from build123d import *

# Parameters (mm, degrees)
BOSS_EXTRUDE1_DEPTH     = 7.75
CUT_EXTRUDE_THIN1_DEPTH = 42.810913647
CUT_EXTRUDE1_REACH      = 43.811
SKETCH3_W               = 7.8
SKETCH3_H               = 2.7
CHAMFER1_SIZE           = 0.5


with BuildPart() as part:
    # Sketch1 → Boss-Extrude1 (new, symmetric)
    with BuildSketch(Plane(origin=(0, 0, 0), x_dir=(0, 0, -1), z_dir=(1, 0, 0))):
        Polygon((0, 0), (40.3, 0), (40.3, 8), (38.3, 8), (38.3, 3.5), (19, 3.5), (19, 1.7), (14, 1.7), (14, 3.5), (9.6, 3.5), (9.6, 2.5), (3, 2.5), (3, 5.2), (1, 5.2), (1, 6.7), (0, 6.7), align=None)
    extrude(amount=BOSS_EXTRUDE1_DEPTH, both=True)

    # Sketch2 → Cut-Extrude-Thin1 (cut, through all)
    with BuildSketch(Plane(origin=(0, 0, 0), x_dir=(1, 0, 0), z_dir=(0, 1, 0))):
        Polygon((-17.75, -10), (17.75, -10), (17.75, 11), (16.25, 11), (16.25, 13), (15, 13), (15, 50.3), (-15, 50.3), (-15, 13), (-16.25, 13), (-16.25, 11), (-17.75, 11), align=None)
        Polygon((-7.75, 0), (7.75, 0), (7.75, 1), (6.25, 1), (6.25, 3), (5, 3), (5, 40.3), (-5, 40.3), (-5, 3), (-6.25, 3), (-6.25, 1), (-7.75, 1), align=None, mode=Mode.SUBTRACT)
    extrude(amount=CUT_EXTRUDE_THIN1_DEPTH, mode=Mode.SUBTRACT)

    # Sketch3 → Cut-Extrude1 (cut, up to next)
    with BuildSketch(Plane.XY, mode=Mode.PRIVATE) as cut_extrude1_sk1:
        with Locations((0, 3.85)):
            Rectangle(SKETCH3_W, SKETCH3_H)
    cut_extrude1_tool1 = extrude(cut_extrude1_sk1.sketch, amount=-CUT_EXTRUDE1_REACH, mode=Mode.PRIVATE) & part.part
    add(cut_extrude1_tool1.solids().sort_by_distance((0, 3.85, 0))[0], mode=Mode.SUBTRACT)

    # Chamfer1
    chamfer1_edges = [part.edges().sort_by_distance(p)[0] for p in [
        (-3.9, 3.85, 0),
        (0, 2.5, 0),
        (3.9, 3.85, 0),
        (0, 5.2, 0),
        (-7.75, 3.35, 0),
        (0, 6.7, 0),
        (0, 0, 0),
        (7.75, 3.35, 0),
    ]]
    chamfer(chamfer1_edges, length=CHAMFER1_SIZE)


solid = part.part
Input: part model. Units: mm. Frame: model coordinates. A direction names the side the tool comes from. Round coordinates to 2 decimals unless told otherwise and drop trailing zeros. Order: outer loops, then holes, each group sorted by start corner. A loop starts at its lowest first (then second) coordinate and runs counter-clockwise, first axis right, second up.
1. Cut plane C-C, the plane z = -15. Output: boundary loops of the cut face in (x, y), then the cut area to 3 significant figures.
The answers:
outline: (-5, 0) - (5, 0) - (5, 1.7) - (-5, 1.7) - close
area: 17.0 mm2
2. Mould query, pull axis X, two halves, no side actions, for faces 5 (the face through (5, 1, -21)), 6 (the face through (0, 2.5, -5)), 7 (the face through (0, 6, -1)). Classes: released by +X, released by -X, zero draft, split by the parting line, or undercut.
The answers:
face 5: released by +X
face 6: undercut
face 7: zero draft
3. Material intervals for line 1 (Z direction, x = -4.5, y = 3); line 2 (Z direction, x = -0.5, y = 6); line 3 (Y direction, x = -2.5, z = -31), sorted ascending.
The answers:
line 1: z = -40.3 to -19, -14 to -9.6, -3 to 0
line 2: z = -40.3 to -38.3, -1 to 0
line 3: y = 0 to 3.5
4. Cut plane A-A, the plane x = -1.5. Output: boundary loops of the cut face in (y, z).
The answers:
outline: (0, -40.3) - (8, -40.3) - (8, -38.3) - (3.5, -38.3) - (3.5, -19) - (1.7, -19) - (1.7, -14) - (3.5, -14) - (3.5, -9.6) - (2.5, -9.6) - (2.5, -0.5) - (2, 0) - (0.5, 0) - (0, -0.5) - close; (5.2, -1) - (6.7, -1) - (6.7, -0.5) - (6.2, 0) - (5.7, 0) - (5.2, -0.5) - close
5. Set-up query: faces 1 (the face through (-6.25, 3, -2)), 2 (the face through (3.9, 4, -2)), 3 (the face through (0, 1.7, -17)), 4 (the face through (-5, 3, -3)). Return all of +Z, -Z, +X, -X, +Y, -Y with unobstructed straight access to the full face (end or side cutting, diameter ignored); none if empty.
The answers:
face 1: -Z, -X, +Y, -Y
face 2: +Z
face 3: +X, -X, +Y
face 4: -X, +Y
6. Cut plane D-D, the plane z = -23.5. Output: boundary loops of the cut face in (x, y).
The answers:
outline: (-5, 0) - (5, 0) - (5, 3.5) - (-5, 3.5) - close
7. Pin query (flat end, axial travel): P1, Ø2.5, axis at x = -1.5, z = -6, coming from the +Y side; P2, Ø1.2, axis at x = -5.5, y = 3, coming from the -Z side; P3, Ø5, axis at x = -0.5, z = -12, coming from the +Y side; P4, Ø1.4, axis at x = -2, y = 3, coming from the +Z side. Return the tip coordinate at first contact, or that it passes through.
The answers:
P1: stops at y = 2.5
P2: stops at z = -40.3
P3: stops at y = 3.5
P4: stops at z = -0.3
8. Cut plane B-B, the plane y = 1. Output: boundary loops of the cut face in (x, z).
The answers:
outline: (-7.75, -1) - (-6.25, -1) - (-6.25, -3) - (-5, -3) - (-5, -40.3) - (5, -40.3) - (5, -3) - (6.25, -3) - (6.25, -1) - (7.75, -1) - (7.75, -0.5) - (7.25, 0) - (-7.25, 0) - (-7.75, -0.5) - close
